Work out the finished part from the listing and answer in its coordinate system (mm). Face numbers are marked on the shaded views. A direction names the side the tool comes from. Round coordinates to 2 decimals unless told otherwise and drop trailing zeros. Use one line per item in the form item = value.
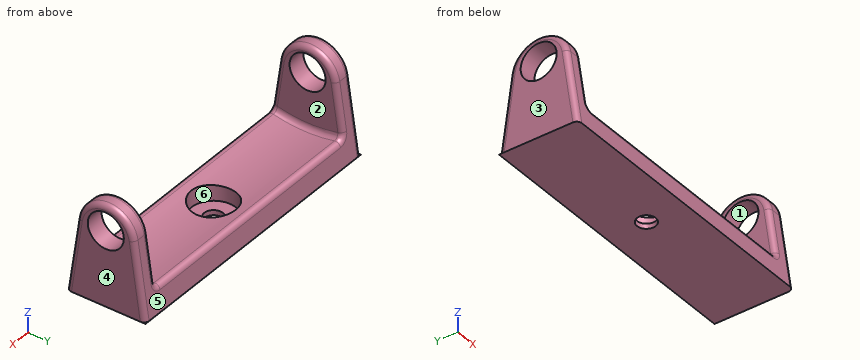
```python
from build123d import *

# Parameters (mm, degrees)
SKETCH_W        = 114.642242
SKETCH_H        = 31.44759
PAD_DEPTH       = 40
POCKET_DEPTH    = 114.643242
SKETCH002_R     = 7.136669
POCKET001_DEPTH = 114.643242
SKETCH003_R     = 55.105675
POCKET002_DEPTH = 50
FILLET_R        = 2
SKETCH004_R     = 8.784385
POCKET003_DEPTH = 7
SKETCH005_R     = 3.710969
POCKET004_DEPTH = 2.001


with BuildPart() as part:
    # Sketch → Pad (new body)
    with BuildSketch(Plane.XY):
        Rectangle(SKETCH_W, SKETCH_H)
    extrude(amount=PAD_DEPTH)

    # Sketch001 (on Face3 of Pad) → Pocket (cut, through all)
    with BuildSketch(Plane.YZ.offset(57.321121)):
        with BuildLine():
            ThreePointArc((11.264383, 29.831773), (-0.014439, 39.554811), (-11.268565, 29.8032))
            Line((-11.268565, 29.8032), (-15.592646, 0))
            Line((-15.592646, 0), (-22.878534, 0))
            Line((-22.878534, 0), (-19.217968, 45.174706))
            Line((-19.217968, 45.174706), (19.051588, 45.174706))
            Line((19.051588, 45.174706), (24.010837, 0))
            Line((15.669825, 0.000428), (24.010837, 0))
            Line((11.264383, 29.831773), (15.669825, 0.000428))
        make_face()
    extrude(amount=-POCKET_DEPTH, mode=Mode.SUBTRACT)

    # Sketch002 (on Face8 of Pocket) → Pocket001 (cut, through all)
    with BuildSketch(Plane.YZ.offset(57.321121)):
        with Locations((0, 29.72154)):
            Circle(SKETCH002_R)
    extrude(amount=-POCKET001_DEPTH, mode=Mode.SUBTRACT)

    # Sketch003 → Pocket002 (cut, symmetric)
    with BuildSketch(Plane.YZ):
        with Locations((0, 62.972816)):
            Circle(SKETCH003_R)
    extrude(amount=POCKET002_DEPTH, both=True, mode=Mode.SUBTRACT)

    # Fillet
    fillet_edges = [part.edges().sort_by_distance(p)[0] for p in [
        (57.321121, -13.430606, 14.9016),
        (57.321121, -0.014439, 39.554811),
        (57.321121, 13.467104, 14.916101),
        (-57.321121, -13.430606, 14.9016),
        (-57.321121, -0.014439, 39.554811),
        (-57.321121, 13.467104, 14.916101),
        (50, 0.025916, 7.867147),
        (0, -14.181911, 9.72332),
        (0, 14.231991, 9.736683),
        (50, -12.725238, 19.76326),
        (50, -0.014439, 39.554811),
        (50, 12.748187, 19.784228),
        (-50, 12.748187, 19.784228),
        (-50, -0.014439, 39.554811),
        (-50, -12.725238, 19.76326),
        (-50, 0.025916, 7.867147),
    ]]
    fillet(fillet_edges, radius=FILLET_R)

    # Sketch004 → Pocket003 (cut)
    with BuildSketch(Plane.XY.offset(9)):
        Circle(SKETCH004_R)
    extrude(amount=-POCKET003_DEPTH, mode=Mode.SUBTRACT)

    # Sketch005 (on Face36 of Pocket003) → Pocket004 (cut, through all)
    with BuildSketch(Plane.XY.offset(2)):
        Circle(SKETCH005_R)
    extrude(amount=-POCKET004_DEPTH, mode=Mode.SUBTRACT)


solid = part.part
```
(1) Consider L1, parallel to X at y = 5, z = 20; L2, parallel to Z at x = 54, y = 0; L3, parallel to X at y = 0, z = 7.5. Determine where each line is inside the solid, lowest interval first.
Completed:
L1 = -57.32 to -50, 50 to 57.32
L2 = 0 to 22.58, 36.86 to 39.55
L3 = -57.32 to -8.78, 8.78 to 57.32
(2) Find section B-B, the plane y = 0. State how many separate pieces and enclosed holes the cut face has, then the cut area to 3 significant figures.
Completed:
separate_pieces = 4
enclosed_holes = 0
area = 1,040 mm2
(3) Given P1, Ø14, axis at x = 4, y = -2.5, coming from the +Z side; P2, Ø10, axis at x = -37, y = -7, coming from the +Z side; P3, Ø1.7, axis at x = -27, y = 15, coming from the +Z side, each flat-ended and moving along its own axis, determine where each tip first touches the part or whether it passes through.
Completed:
P1 = 8.69
P2 = 9.19
P3 = 8.5
(4) For the marked faces 5 and 6, determine the directions among +Z, -Z, +X, -X, +Y, -Y from which every point of the face is accessible in a straight line to the end or side of a thin tool.
Completed:
face_5 = +Z, +X, -X, +Y
face_6 = +Z
(5) For a pull along X with two mould halves and no side action, classify the marked faces 1, 2, 3 and 4 as +X half, -X half, draft (parallel to the pull), parting line (faces both ways), or undercut.
Completed:
face_1 = draft
face_2 = undercut
face_3 = -X half
face_4 = +X half
